Work out the finished part from the listing and answer in its coordinate system (mm). Face numbers are marked on the shaded views. A direction names the side the tool comes from. Round coordinates to 2 decimals unless told otherwise and drop trailing zeros. Order: outer loops, then holes, each group sorted by start corner. A loop starts at its lowest first (then second) coordinate and runs counter-clockwise, first axis right, second up. Notation, with made-up numbers: M 70.5,2 L 104.5,2 A26 ccw 104.5,40 Z; hole C 25,23 d8. An arc over 180 degrees is marked long. Return JSON: item names as keys, results as strings.
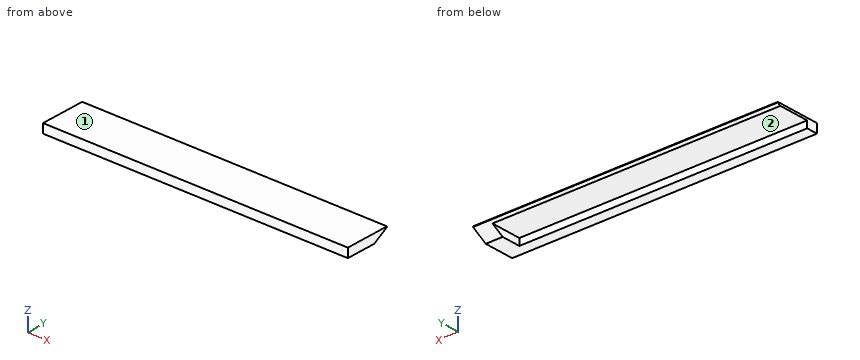
from build123d import *

# Parameters (mm, degrees)
SKETCH_1_W      = 54
SKETCH_1_H      = 8
EXTRUDE_1_DEPTH = 0.4
SKETCH_2_W      = 3
SKETCH_2_H      = 8
EXTRUDE_2_DEPTH = 1.2
SKETCH_3_W      = 54
SKETCH_3_H      = 1.6
EXTRUDE_3_DEPTH = 2
CHAMFER_1_SIZE  = 1.5
CHAMFER_1_SIZE2 = 2.598076211


with BuildPart() as part:
    # 草图1 → 凸台-拉伸1 (new body)
    with BuildSketch(Plane.XY):
        Rectangle(SKETCH_1_W, SKETCH_1_H)
    extrude(amount=EXTRUDE_1_DEPTH)

    # 草图2 → 凸台-拉伸2 (add)
    with BuildSketch(Plane(origin=(0, 0, 0), x_dir=(-1, 0, 0), z_dir=(0, 0, -1))):
        with Locations((-25.5, 0)):
            Rectangle(SKETCH_2_W, SKETCH_2_H)
    extrude(amount=EXTRUDE_2_DEPTH)

    # 草图3 → 凸台-拉伸3 (add)
    with BuildSketch(Plane.XZ.offset(4)):
        with Locations((0, -0.4)):
            Rectangle(SKETCH_3_W, SKETCH_3_H)
    extrude(amount=-EXTRUDE_3_DEPTH)

    # 倒角1
    chamfer_1_edges = [part.edges().sort_by_distance(p)[0] for p in [
        (25.5, 4, -1.2),
    ]]
    chamfer_1_side = [part.faces().sort_by_distance(p)[0] for p in [
        (3.642857143, 4, 0.085714286),
    ]]
    chamfer(chamfer_1_edges, length=CHAMFER_1_SIZE, length2=CHAMFER_1_SIZE2, reference=chamfer_1_side[0])


solid = part.part
Item 1: Find section A-A (x = -18). Determine the outline of the cut face in (y, z), plus the area to 3 significant figures.
Output:
{"outline": "M -4,-1.2 L -2,-1.2 L -2,0 L 3.48,0 L 4,0.3 L 4,0.4 L -4,0.4 Z", "area": "5.52 mm^2"}
Item 2: Consider line 1 along Z through (x, y) = (-14.5, 2.25); line 2 along X through (y, z) = (1.5, -0.25); line 3 along Y through (x, z) = (-23, -0.65). Determine where each line is inside the solid, lowest interval first. Write a range as [from, to].
Output:
{"line 1": "z = [0, 0.4]", "line 2": "x = [24, 27]", "line 3": "y = [-4, -2]"}
Item 3: Find section B-B (y = -1.5). Determine the outline of the cut face in (x, z), plus the area to 3 significant figures.
Output:
{"outline": "M -27,0 L 24,0 L 24,-1.2 L 27,-1.2 L 27,0.4 L -27,0.4 Z", "area": "25.2 mm^2"}
Item 4: Which of the six approach directions +Z, -Z, +X, -X, +Y, -Y give full straight-line access (tool end or side, diameter ignored) to the marked faces 1 and 2?
Output:
{"face 1": "+Z, +X, -X, +Y, -Y", "face 2": "-Z, -X, +Y"}
Item 5: Find section C-C (z = -0.45). Determine the outline of the cut face in (x, y), plus the area to 3 significant figures.
Output:
{"outline": "M -27,-4 L 27,-4 L 27,2.7 L 24,2.7 L 24,-2 L -27,-2 Z", "area": "122 mm^2"}
Item 6: This flat-tipped pin is pushed along its axis until it touches: pin 1 (4.5 mm diameter, centred on x = -1, y = 2, fed in from -Z). Where does it stop, or does it pass through?
Output:
{"pin 1": "stops at z = 0"}
